from build123d import *

# Parameters (mm, degrees)
SKETCH1_W           = 80
SKETCH1_H           = 36
BOSS_EXTRUDE1_DEPTH = 1.6
SKETCH2_R           = 1.25
CUT_EXTRUDE1_DEPTH  = 1.6
SKETCH3_W           = 71
SKETCH3_H           = 25
BOSS_EXTRUDE2_DEPTH = 8.5
SKETCH4_R           = 0.261136338
BOSS_EXTRUDE3_DEPTH = 0.1
LPATTERN1_COUNT     = 16
LPATTERN1_PITCH     = 2.54


with BuildPart() as part:
    # Sketch1 → Boss-Extrude1 (new body)
    with BuildSketch(Plane(origin=(0, 0, 0), x_dir=(1, 0, 0), z_dir=(0, 1, 0))):
        Rectangle(SKETCH1_W, SKETCH1_H)
    extrude(amount=BOSS_EXTRUDE1_DEPTH)

    # Sketch2 → Cut-Extrude1 (cut)
    with BuildSketch(Plane(origin=(0, 1.6, 0), x_dir=(1, 0, 0), z_dir=(0, 1, 0))):
        with Locations(Location((-37.5, 15.5, 0), (0, 0, 270))):
            Circle(SKETCH2_R)
        with Locations(Location((37.5, 15.5, 0), (0, 0, 270))):
            Circle(SKETCH2_R)
        with Locations(Location((37.5, -15.5, 0), (0, 0, 270))):
            Circle(SKETCH2_R)
        with Locations(Location((-37.5, -15.5, 0), (0, 0, 270))):
            Circle(SKETCH2_R)
    extrude(amount=-CUT_EXTRUDE1_DEPTH, mode=Mode.SUBTRACT)

    # Sketch3 → Boss-Extrude2 (add)
    with BuildSketch(Plane(origin=(0, 1.6, 0), x_dir=(1, 0, 0), z_dir=(0, 1, 0))):
        Rectangle(SKETCH3_W, SKETCH3_H)
    extrude(amount=BOSS_EXTRUDE2_DEPTH)

    # Sketch4 → Boss-Extrude3 (add)
    with BuildSketch(Plane(origin=(0, 1.6, 0), x_dir=(1, 0, 0), z_dir=(0, 1, 0))):
        with BuildLine():
            Line((-33, 16), (-33, 18))
            Line((-33, 18), (-31, 18))
            Line((-31, 18), (-31, 16))
            ThreePointArc((-31, 16), (-32, 15), (-33, 16))
        make_face()
        with Locations(Location((-32, 16, 0), (0, 0, 270))):
            Circle(SKETCH4_R, mode=Mode.SUBTRACT)
    boss_extrude3 = extrude(amount=BOSS_EXTRUDE3_DEPTH)

    # LPattern1: Boss-Extrude3 ×16
    with Locations(*[(i * LPATTERN1_PITCH, 0, 0) for i in range(1, LPATTERN1_COUNT)]):
        add(boss_extrude3)


solid = part.part
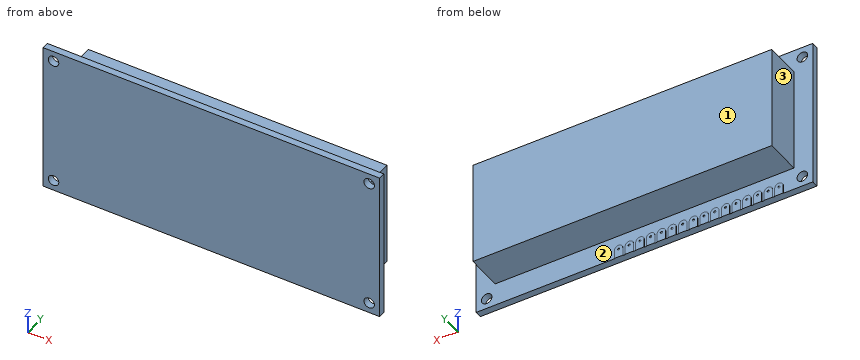
Source: CAD feature listing. Evaluate the final solid. Frame: model axes, mm. Face numbers are marked on the shaded views. A direction names the side the tool comes from. Round coordinates to 2 decimals unless told otherwise and drop trailing zeros. Loops run counter-clockwise (first coordinate to the right, second up) from the corner with the lowest first, then second, coordinate; pieces in that order, holes last.
Q1. Section B-B, the plane z = -7. Return loops of the section in (x, y), plus the area to 4 significant figures.
Q2. Section A-A, the plane z = 15.5. Return loops of the section in (x, y), plus the area to 3 significant figures.
Q3. Section D-D, the plane y = 6.5. Return loops of the section in (x, z).
Q4. Access query for the marked faces 1, 2 and 3. Directions: +Z, -Z, +X, -X, +Y, -Y. A direction counts if a zero-diameter tool reaches every point of the face in a straight line with its end or side. Return the directions, or none.
Q5. First-contact query: P1, Ø1, axis at x = -8.5, y = 2, coming from the -Z side; P2, Ø0.6, axis at x = -1.5, z = -16, coming from the +Y side; P3, Ø1.5, axis at x = -8, y = 3, coming from the +Z side; P4, Ø1.5, axis at x = -8, y = 8.5, coming from the -Z side. Flat tips, straight axial feed; report the tip coordinate or a pass-through.
Q6. Ray query, line 1 (X direction, y = 0.8, z = -15.5); line 2 (X direction, y = 6.75, z = -10.5); line 3 (Z direction, x = -1.52, y = 1.75). Return the intervals inside material, ascending.
Q7. Section C-C, the plane x = 8. Return loops of the section in (y, z), plus the area to 3 significant figures.
Solutions:
1. outline: (-40, 0) - (40, 0) - (40, 1.6) - (35.5, 1.6) - (35.5, 10.1) - (-35.5, 10.1) - (-35.5, 1.6) - (-40, 1.6) - close
1. area: 731.5 mm2
2. outline: (-40, 0) - (-38.75, 0) - (-38.75, 1.6) - (-40, 1.6) - close; (-36.25, 0) - (36.25, 0) - (36.25, 1.6) - (-36.25, 1.6) - close; (38.75, 0) - (40, 0) - (40, 1.6) - (38.75, 1.6) - close
2. area: 120 mm2
3. outline: (-35.5, -12.5) - (35.5, -12.5) - (35.5, 12.5) - (-35.5, 12.5) - close
4. face 1: +Z, -Z, +X, -X, +Y
4. face 2: +Y
4. face 3: +Z, -Z, -X, +Y
5. P1: stops at z = -18
5. P2: stops at y = 1.7
5. P3: stops at z = 12.5
5. P4: stops at z = -12.5
6. line 1: x = -40 to -38.75, -36.25 to 36.25, 38.75 to 40
6. line 2: x = -35.5 to 35.5
6. line 3: z = -12.5 to 12.5
7. outline: (0, -18) - (1.6, -18) - (1.6, -12.5) - (10.1, -12.5) - (10.1, 12.5) - (1.6, 12.5) - (1.6, 18) - (0, 18) - close
7. area: 270 mm2
